Geometry: final body of the model. Coordinates: model frame, mm. A direction names the side the tool comes from. Coordinates: 2 decimals unless noted, no trailing zeros. Order: outer loops, then holes, each group sorted by start corner. A loop starts at its lowest first (then second) coordinate and runs counter-clockwise, first axis right, second up. Notation, with made-up numbers: (22.25, -26.75) -> (77.25, -26.75) arc R24 ccw to (77.25, 0.25) -> close; hole circle Ø6 at (45.25, 12). An arc over 180 degrees is marked (long way). Use CSV: the item, a comma, the result in double quotes. Start each with the question number.
Autodesk Inventor part; units mm, degrees
ref_plane "YZ Plane" through (0, 0, 0) normal (1, 0, 0) x (0, 1, 0)
ref_plane "XZ Plane" through (0, 0, 0) normal (0, 1, 0) x (-1, 0, 0)
ref_plane "XY Plane" through (0, 0, 0) normal (0, 0, 1) x (1, 0, 0)
sketch "Sketch1" plane through (0, 0, 0) normal (0, 0, 1) x (1, 0, 0)
  line L0 (0, 0) -> (30, 0)
  line L1 (0, 0) -> (-12.1809, 20.6791)
  line L2 (0, 0) -> (24, 0) construction
  line L3 (-12.1809, 20.6791) -> (-6.1495, 24.2319)
  line L4 (30, 0) -> (30, 2)
  line L5 (30, 2) -> (6.9461, 2)
  line L6 (6.9461, 2) -> (-6.1495, 24.2319)
  dimension "d0" = 30
  dimension "d1" = 24
  dimension "d2" = 120.5
  dimension "d3" = 7
  dimension "d4" = 2
extrude "Extrusion1" add sketch "Sketch1" along normal blind 30
sketch "Sketch2" plane through (-12.1809, 20.6791, 30) normal (-0.5075384, 0.8616292, 0) x (0.8616292, 0.5075384, 0)
  line L0 (1.75, 26) -> (5.25, 26)
  line L1 (5.25, 26) -> (5.25, 4)
  line L2 (5.25, 4) -> (1.75, 4)
  line L3 (1.75, 4) -> (1.75, 26)
  line L4 (7, 30) -> (7, 0)
  line L5 (0, 30) -> (0, 0)
  line L6 (7, 0) -> (0, 0)
  line L7 (7, 30) -> (0, 30)
  dimension "d7" = 22
  dimension "d8" = 3.5
  dimension "d9" = 7
  dimension "d10" = 30
  dimension "d11" = 4
  dimension "d12" = 1.75
extrude "Extrusion2" cut sketch "Sketch2" against normal through all contours L0 L1 L2 L3
sketch "Sketch3" plane through (0, 0, 0) normal (-0.8616292, -0.5075384, 0) x (0, 0, 1)
  circle A0 centre (15, 10) radius 6.5
  line L0 (30, 24) -> (30, 0)
  line L1 (0, 24) -> (0, 0)
  line L2 (0, 24) -> (30, 24)
  dimension "d15" = 13
  dimension "d16" = 30
  dimension "d17" = 15
  dimension "d18" = 14
extrude "Extrusion3" cut sketch "Sketch3" against normal through all
equation "\"d11\" = -0.5 * d7 + 0.5 * d10"
equation "\"d12\" = -0.5 * d8 + 0.5 * d9"
equation "\"d17\" = 0.5 * d16"
properties part number "vtail_wing_piece"
(1) Line query: line 1 (Y direction, x = 27, z = 27.5); line 2 (X direction, y = 4.75, z = 22.75); line 3 (Z direction, x = 2, y = 9.25). Output: solid intervals per line, ascending. Write a range as from..to.
(2) First-contact query: pin 1 (12 mm diameter, centred on y = 16, z = 8, fed in from +X); pin 2 (11.5 mm diameter, centred on x = 22, z = 15.5, fed in from +Y); pin 3 (2 mm diameter, centred on y = 6, z = 14.5, fed in from +X). Flat tips, straight axial feed; report the tip coordinate or a pass-through.
(3) Access query for faces 1 (the face through (19, 2, 15)), 2 (the face through (-2, 11, 4)), 3 (the face through (-8.71, 14.79, 14.79)). Directions: +Z, -Z, +X, -X, +Y, -Y. A direction counts if a zero-diameter tool reaches every point of the face in a straight line with its end or side. Return the directions, or none.
(4) Section D-D (x = 5.5). Return loops of the section in (y, z).
(5) Section C-C (z = 27.5). Return loops of the section in (x, y).
(6) Section A-A (z = 24.5). Return loops of the section in (x, y).
(7) Mould query, pull axis Z, two halves, no side actions, for faces 4 (the face through (1, 9, 0)), 5 (the face through (-2, 11, 26)), 6 (the face through (15, 0, 15)). Classes: pulls with the +Z half, pulls with the -Z half, needs draft (parallel to the pull), parting line crosses it, or undercut.
(8) Section B-B (y = 19.75). Return loops of the section in (x, z), then the cut area to 3 significant figures.
Check sheet entries:
1,line 1,"y = 0..2"
1,line 2,"x = -2.8..-0.77, 3.3..5.33"
1,line 3,"z = 0..9.26, 20.74..30"
2,pin 1,"stops at x = 2.23"
2,pin 2,"stops at y = 2"
2,pin 3,"stops at x = 5.18"
3,face 1,"+Z, -Z, +X, +Y"
3,face 2,"none"
3,face 3,"+Z, -Z, -X, -Y"
4,outline,"(0, 0) -> (4.45, 0) -> (4.45, 30) -> (0, 30) -> (0, 26) -> (1.01, 26) -> (1.01, 4) -> (0, 4) -> close"
5,outline,"(-12.18, 20.68) -> (0, 0) -> (30, 0) -> (30, 2) -> (6.95, 2) -> (-6.15, 24.23) -> close"
6,outline,"(-12.18, 20.68) -> (0, 0) -> (2.03, 0) -> (-10.67, 21.57) -> close; (-7.66, 23.34) -> (6.09, 0) -> (30, 0) -> (30, 2) -> (6.95, 2) -> (-6.15, 24.23) -> close"
7,face 4,"pulls with the -Z half"
7,face 5,"undercut"
7,face 6,"needs draft"
8,outline,"(-11.63, 0) -> (-3.51, 0) -> (-3.51, 30) -> (-11.63, 30) -> close; hole (-9.6, 4) -> (-5.54, 4) -> (-5.54, 26) -> (-9.6, 26) -> close"
8,area,"154 mm^2"
